Part model, mm, in its own coordinate system. A direction names the side the tool comes from. Round coordinates to 2 decimals unless told otherwise and drop trailing zeros. Order: outer loops, then holes, each group sorted by start corner. A loop starts at its lowest first (then second) coordinate and runs counter-clockwise, first axis right, second up. Notation, with made-up numbers: M 51,-39 L 90,-39 A22 cw 90,-29 Z; hole C -36.5,-31.5 d8. An arc over 180 degrees is marked long. Write each question's results on one line, items separated by ' | '. Start each with the question number.
1. Band-saw the part on C-C, the plane z = 60. List the corners of the cut face in (x, y).
2. Which spindle directions (+Z, -Z, +X, -X, +Y, -Y) get a long thin tool onto all of the face, cutting with end or side? Do faces 1 (the face through (-45.5, -39.3, 54.2)), 2 (the face through (64, -3, 109)), 3 (the face through (74.92, -2.72, 108.5)). Say none if no direction does.
3. Probe L1, parallel to X at y = -41, z = 54.5; L2, parallel to X at y = 16, z = 104.5; L3, parallel to X at y = -35, z = 42.5. List the from-to ranges inside material, lowest first. Write a range as [from, to].
4. Drop flat-ended pins along their axis: pin 1 Ø12 at (x, y) = (-34, -30.5) entering from -Z; pin 2 Ø15.5 at (x, y) = (61, 0) entering from -Z; pin 3 Ø1 at (x, z) = (-57, 93) entering from -Y; pin 4 Ø1.5 at (x, z) = (27, 56) entering from -Y. Give the stop position or say it passes through.
5. Two-plate mould, pull along Y, no slides. Class faces 4 (the face through (75.348, -3, 52)), 5 (the face through (-74.146, 52.078, 54.23)), 6 (the face through (-74.92, 52.72, 54.23)), 7 (the face through (76, -53.219, 55)): +Y half, -Y half, draft (parallel to the pull), parting line (faces both ways), or undercut.
6. Band-saw the part on B-B, the plane y = -6. List the corners of the cut face in (x, z).
7. Band-saw the part on A-A, the plane x = 63. List the corners of the cut face in (y, z), then the cut area to 3 significant figures.
8. Band-saw the part on D-D, the plane x = -44. List the corners of the cut face in (y, z).
```python
from build123d import *

# Parameters (mm, degrees)
BASE_FLANGE1_DEPTH           = 110
EDGE_FLANGE1_DEPTH           = 110
EDGE_FLANGE1_2_DEPTH         = 110
EDGE_FLANGE2_STRIP_W         = 12
EDGE_FLANGE2_STRIP_H         = 1
EDGE_FLANGE2_STRIP_CUT_DEPTH = 102.437324841
EDGE_FLANGE2_DEPTH           = 102.437324841


# Read off the part's stored shape, not the designer's step: Edge-Flange1
# Sheet-metal steps are written as plain solids
with BuildPart() as part:
    # Sketch1 → Base-Flange1 (new body)
    with BuildSketch(Plane.XY):
        with BuildLine():
            Line((75.34839628, -53.21866242), (75.34839628, 49.21866242))
            ThreePointArc((75.34839628, 49.21866242), (74.176823405, 52.047089545), (71.34839628, 53.21866242))
            Line((71.34839628, 53.21866242), (-71.34839628, 53.21866242))
            ThreePointArc((-71.34839628, 53.21866242), (-74.176823405, 52.047089545), (-75.34839628, 49.21866242))
            Line((-75.34839628, 49.21866242), (-75.34839628, -53.21866242))
            Line((-75.34839628, -53.21866242), (-76.34839628, -53.21866242))
            Line((-76.34839628, -53.21866242), (-76.34839628, 49.21866242))
            ThreePointArc((-76.34839628, 49.21866242), (-74.883930186, 52.754196326), (-71.34839628, 54.21866242))
            Line((-71.34839628, 54.21866242), (71.34839628, 54.21866242))
            ThreePointArc((71.34839628, 54.21866242), (74.883930186, 52.754196326), (76.34839628, 49.21866242))
            Line((76.34839628, 49.21866242), (76.34839628, -53.21866242))
            Line((76.34839628, -53.21866242), (75.34839628, -53.21866242))
        make_face()
    extrude(amount=BASE_FLANGE1_DEPTH)

    # Edge-Flange1 outline → Edge-Flange1 (cut)
    with BuildSketch(Plane.XY):
        with BuildLine():
            Line((-75.34839628, -53.21866242), (-75.34839628, -48.836542193))
            ThreePointArc((-75.34839628, -48.836542193), (-76.09181277, -47.417681023), (-76.34839628, -45.836542193))
            Line((-76.34839628, -45.836542193), (-76.34839628, -53.21866242))
            Line((-76.34839628, -53.21866242), (-75.34839628, -53.21866242))
        make_face()
    extrude(amount=EDGE_FLANGE1_DEPTH, mode=Mode.SUBTRACT)

    # Edge-Flange1 2 outline → Edge-Flange1 2 (add)
    with BuildSketch(Plane.XY):
        with BuildLine():
            ThreePointArc((-75.34839628, -48.836542193), (-72.563513138, -50.686644359), (-69.235304971, -50.368081128))
            Line((-69.235304971, -50.368081128), (-21.063621271, -27.905256112))
            Line((-21.063621271, -27.905256112), (-21.486239533, -26.998948325))
            Line((-21.486239533, -26.998948325), (-69.657923233, -49.461773341))
            ThreePointArc((-69.657923233, -49.461773341), (-73.497594713, -49.210107976), (-75.34839628, -45.836542193))
            Line((-75.34839628, -45.836542193), (-75.34839628, -48.836542193))
        make_face()
    extrude(amount=EDGE_FLANGE1_2_DEPTH)

    # Edge-Flange2 strip (across the edge) → Edge-Flange2 strip cut (cut)
    with BuildSketch(Plane(origin=(75.34839628, -53.21866242, 110), x_dir=(0, 0, -1), z_dir=(0, 1, 0))):
        with Locations((-1, -0.5)):
            Rectangle(EDGE_FLANGE2_STRIP_W, EDGE_FLANGE2_STRIP_H)
    extrude(amount=EDGE_FLANGE2_STRIP_CUT_DEPTH, mode=Mode.SUBTRACT)

    # Edge-Flange2 section (across the edge) → Edge-Flange2 (add)
    with BuildSketch(Plane(origin=(75.34839628, -53.21866242, 110), x_dir=(0, 0, -1), z_dir=(0, 1, 0))):
        with BuildLine():
            Line((0, 4), (0, 18))
            Line((0, 18), (1, 18))
            Line((1, 18), (1, 4))
            ThreePointArc((1, 4), (2.171572875, 1.171572875), (5, 0))
            Line((5, 0), (5, -1))
            ThreePointArc((5, -1), (1.464466094, 0.464466094), (0, 4))
        make_face()
    extrude(amount=EDGE_FLANGE2_DEPTH)


solid = part.part
```
Solution:
1) outline: M -76.35,-45.84 A5 ccw -69.24,-50.37 L -21.06,-27.91 L -21.49,-27 L -69.66,-49.46 A4 cw -75.35,-45.84 L -75.35,49.22 A4 cw -71.35,53.22 L 71.35,53.22 A4 cw 75.35,49.22 L 75.35,-53.22 L 76.35,-53.22 L 76.35,49.22 A5 ccw 71.35,54.22 L -71.35,54.22 A5 ccw -76.35,49.22 Z
2) face 1: +Z, -Z, -Y | face 2: -Z, -Y | face 3: +Z, +X, -Y
3) L1: [-76.35, -75.35], [-51.51, -49.15], [75.35, 76.35] | L2: [-76.35, -75.35], [75.35, 76.35] | L3: [-76.35, -75.35], [-38.64, -36.28], [75.35, 76.35]
4) pin 1: z = 0 | pin 2: z = 109 | pin 3: y = -44.9 | pin 4: y = 53.22
5) face 4: draft | face 5: undercut | face 6: +Y half | face 7: -Y half
6) outline: M -76.35,0 L -75.35,0 L -75.35,110 L -76.35,110 Z; M 57.35,109 L 71.35,109 A4 cw 75.35,105 L 75.35,0 L 76.35,0 L 76.35,105 A5 ccw 71.35,110 L 57.35,110 Z
7) outline: M -53.22,109 L 49.22,109 L 49.22,110 L -53.22,110 Z; M 53.22,0 L 54.22,0 L 54.22,110 L 53.22,110 Z | area: 212 mm^2
8) outline: M -38.6,0 L -37.5,0 L -37.5,110 L -38.6,110 Z; M 53.22,0 L 54.22,0 L 54.22,110 L 53.22,110 Z
